from build123d import *

# Parameters (mm, degrees)
SKETCH_1_W          = 35
SKETCH_1_H          = 43.5
EXTRUDE_1_DEPTH     = 20
SKETCH_2_W          = 20
SKETCH_2_H          = 5
EXTRUDE_2_DEPTH     = 10
SKETCH_3_W          = 20
SKETCH_3_H          = 5
EXTRUDE_3_DEPTH     = 10
SKETCH_4_R          = 1.5
CUT_EXTRUDE_2_DEPTH = 5
SKETCH_5_R          = 11.25
CUT_EXTRUDE_4_DEPTH = 20


with BuildPart() as part:
    # Эскиз1 → Бобышка-Вытянуть1 (new body)
    with BuildSketch(Plane.XY):
        Rectangle(SKETCH_1_W, SKETCH_1_H)
    extrude(amount=EXTRUDE_1_DEPTH)

    # Эскиз2 → Бобышка-Вытянуть2 (add)
    with BuildSketch(Plane(origin=(17.5, 0, 0), x_dir=(0, 0, -1), z_dir=(1, 0, 0))):
        with Locations((-10, -19.25)):
            Rectangle(SKETCH_2_W, SKETCH_2_H)
    extrude(amount=EXTRUDE_2_DEPTH)

    # Эскиз3 → Бобышка-Вытянуть3 (add)
    with BuildSketch(Plane.ZY.offset(17.5)):
        with Locations((10, -19.25)):
            Rectangle(SKETCH_3_W, SKETCH_3_H)
    extrude(amount=EXTRUDE_3_DEPTH)

    # Эскиз4 → Вырез-Вытянуть2 (cut)
    with BuildSketch(Plane(origin=(0, -16.75, 0), x_dir=(1, 0, 0), z_dir=(0, 1, 0))):
        with Locations((-22.5, -16)):
            Circle(SKETCH_4_R)
        with Locations((-22.5, -4)):
            Circle(SKETCH_4_R)
        with Locations((22.5, -16)):
            Circle(SKETCH_4_R)
        with Locations((22.5, -4)):
            Circle(SKETCH_4_R)
    extrude(amount=-CUT_EXTRUDE_2_DEPTH, mode=Mode.SUBTRACT)

    # Эскиз5 → Вырез-Вытянуть4 (cut)
    with BuildSketch(Plane(origin=(0, 0, 0), x_dir=(-1, 0, 0), z_dir=(0, 0, -1))):
        with Locations((0, 8.25)):
            Circle(SKETCH_5_R)
    extrude(amount=-CUT_EXTRUDE_4_DEPTH, mode=Mode.SUBTRACT)


solid = part.part
Verification items for the finished model (mm, model axes). A direction names the side the tool comes from. Coordinates: 2 decimals unless noted, no trailing zeros. Write each loop counter-clockwise with the first axis right and the second up, starting at its lowest first coordinate (ties: lowest second). Pieces come first, ordered by that corner, then holes. Notation, with made-up numbers: M -33,2.25 L -24,2.25 A27 ccw -24,18.25 Z; hole C 34.25,-35 d5. An arc over 180 degrees is marked long. Use a Markdown table: item, result.
Q1. Draft check along Z on faces 1 (the face through (0, -5, 20)), 2 (the face through (21, -19, 4)), 3 (the face through (0, -21.75, 10)). Enter one of: +Z half, -Z half, draft (parallel to the pull), parting line (faces both ways), or undercut.
Reply:
| item | result |
|---|---|
| face 1 | +Z half |
| face 2 | undercut |
| face 3 | draft |
Q2. Sectioned sample at D-D, the plane x = -22.5. Record the boundary of the cut face in (y, z).
Reply:
| item | result |
|---|---|
| outline | M -21.75,0 L -16.75,0 L -16.75,2.5 L -21.75,2.5 Z; M -21.75,5.5 L -16.75,5.5 L -16.75,14.5 L -21.75,14.5 Z; M -21.75,17.5 L -16.75,17.5 L -16.75,20 L -21.75,20 Z |
Q3. Sectioned sample at A-A, the plane z = 16. Record the boundary of the cut face in (x, y).
Reply:
| item | result |
|---|---|
| outline | M -27.5,-21.75 L -24,-21.75 L -24,-16.75 L -27.5,-16.75 Z; M -21,-21.75 L 21,-21.75 L 21,-16.75 L 17.5,-16.75 L 17.5,21.75 L -17.5,21.75 L -17.5,-16.75 L -21,-16.75 Z; M 24,-21.75 L 27.5,-21.75 L 27.5,-16.75 L 24,-16.75 Z; hole C 0,8.25 d22.5 |
Q4. Sectioned sample at B-B, the plane x = 0. Record the boundary of the cut face in (y, z).
Reply:
| item | result |
|---|---|
| outline | M -21.75,0 L -3,0 L -3,20 L -21.75,20 Z; M 19.5,0 L 21.75,0 L 21.75,20 L 19.5,20 Z |
Q5. Set-up check for faces 4 (the face through (-17.5, 2, 10)), 5 (the face through (-27.5, -19, 10)), 6 (the face through (17.5, 2, 10)): record each of +Z, -Z, +X, -X, +Y, -Y from which the full face is reachable in a straight line by a thin tool's end or side.
Reply:
| item | result |
|---|---|
| face 4 | +Z, -Z, -X, +Y |
| face 5 | +Z, -Z, -X, +Y, -Y |
| face 6 | +Z, -Z, +X, +Y |
Q6. Go/stop test with flat-tipped pins: P1, Ø2, axis at x = 20, y = 11, coming from the +Z side; P2, Ø3.5, axis at x = -22.5, z = 16, coming from the +Y side; P3, Ø6, axis at y = 0, z = 10.5, coming from the -X side; P4, Ø6, axis at y = 11, z = 6, coming from the +X side. Record where each tip stops, or that it passes through.
Reply:
| item | result |
|---|---|
| P1 | passes through |
| P2 | stops at y = -16.75 |
| P3 | stops at x = -17.5 |
| P4 | stops at x = 17.5 |
Q7. Sectioned sample at C-C, the plane z = 10.75. Record the boundary of the cut face in (x, y), plus the area to 3 significant figures.
Reply:
| item | result |
|---|---|
| outline | M -27.5,-21.75 L 27.5,-21.75 L 27.5,-16.75 L 17.5,-16.75 L 17.5,21.75 L -17.5,21.75 L -17.5,-16.75 L -27.5,-16.75 Z; hole C 0,8.25 d22.5 |
| area | 1,220 mm² |
Q8. Thickness scan on line 1 (X direction, y = -19.7, z = 4); line 2 (Z direction, x = -22.5, y = -17.95); line 3 (X direction, y = -7, z = 10). Record the ranges inside material, lowest first.
Reply:
| item | result |
|---|---|
| line 1 | x = -27.5 to -24, -21 to 21, 24 to 27.5 |
| line 2 | z = 0 to 2.5, 5.5 to 14.5, 17.5 to 20 |
| line 3 | x = -17.5 to 17.5 |
